Part model, mm, in its own coordinate system. A direction names the side the tool comes from. Give positions to 0.01 mm unless a question says otherwise; leave off trailing zeros. Order: outer loops, then holes, each group sorted by start corner. A loop starts at its lowest first (then second) coordinate and runs counter-clockwise, first axis right, second up. Notation, with made-up numbers: (-15, 48) -> (37, 48) arc R16 cw to (37, 71) -> close; hole circle Ø4 at (65, 25). An arc over 180 degrees is marked (long way). Write item = value, one per line. Start each with the question number.
Item 1: Band-saw the part on C-C on z = 22.5. Write the cut outline in (x, y).
Item 2: Band-saw the part on D-D on x = 13. Write the cut outline in (y, z), plus the area to 3 significant figures.
Item 3: Band-saw the part on A-A on x = 0. Write the cut outline in (y, z), plus the area to 3 significant figures.
Item 4: Tool access for faces 4 (the face through (9, 20, -12)), 5 (the face through (-18, -18.5, 24)): list every direction of +Z, -Z, +X, -X, +Y, -Y with a clear straight run to the whole face (end or side of a thin tool).
Item 5: Band-saw the part on B-B on y = 0. Write the cut outline in (x, z).
Item 6: Drill centre lines: line 1 along Y through (x, z) = (0, -14); line 2 along Y through (x, z) = (0, -6.25); line 3 along X through (y, z) = (-7.5, 19.5). Where is each one in solid material? Low to high.
Item 7: Flat gauge pins, fed straight in: P1, Ø6, axis at x = -2, y = 9.5, coming from the +Z side; P2, Ø4.5, axis at x = -16, z = 5, coming from the -Y side; P3, Ø9.5, axis at x = 0, y = -24, coming from the -Z side. Where does each tip first touch, or does it go through?
Item 8: Pull direction X, two halves, no side cores. Call faces 1 (the face through (0.1, -27.4, -10)), 2 (the face through (9, -20, -12)), 3 (the face through (-27, -16, -12)): +X half, -X half, draft (parallel to the pull), parting line (faces both ways), or undercut.
```python
from build123d import *

# Parameters (mm, degrees)
SKETCH1_R                = 9
SKETCH1_R_2              = 3
SKETCH1_W                = 32
SKETCH1_H                = 8
BOSS_EXTRUDE1_DEPTH      = 25
BOSS_EXTRUDE2_DEPTH      = 15
BOSS_EXTRUDE3_DEPTH      = 14
SKETCH3_R                = 12.5
BOSS_EXTRUDE4_DEPTH      = 20
BOSS_EXTRUDE5_DEPTH      = 18
SKETCH5_R                = 10
BOSS_EXTRUDE6_DEPTH      = 25
BOSS_EXTRUDE7_REACH      = 103.681
BOSS_EXTRUDE7_END_RADIUS = 10
SKETCH7_W                = 5
SKETCH7_H                = 1
BOSS_EXTRUDE8_DEPTH      = 1
SKETCH7_4_W              = 5
SKETCH7_4_H              = 1
BOSS_EXTRUDE9_DEPTH      = 4
SKETCH10_R               = 8
CUT_EXTRUDE1_DEPTH       = 15


with BuildPart() as part:
    # Sketch1 → Boss-Extrude1 (new body)
    # profile 1 of 4: a face of its own
    with BuildSketch(Plane(origin=(0, 0, 0), x_dir=(0, 1, 0), z_dir=(0, 0, 1))):
        with Locations((-24, 0)):
            Circle(SKETCH1_R)
        with Locations(Location((-24, 0, 0), (0, 0, 270))):
            Circle(SKETCH1_R_2, mode=Mode.SUBTRACT)
    # profile 2 of 4: a face of its own
    with BuildSketch(Plane(origin=(0, 0, 0), x_dir=(0, 1, 0), z_dir=(0, 0, 1))):
        with BuildLine():
            ThreePointArc((-15, 0), (-17.636038969, -6.363961031), (-24, -9))
            Line((-24, -9), (-16, -9))
            Line((-16, -9), (16, -9))
            Line((16, -9), (24, -9))
            ThreePointArc((24, -9), (15, 0), (24, 9))
            Line((24, 9), (24, 21))
            Line((24, 21), (8, 33))
            Line((8, 33), (-8, 33))
            Line((-8, 33), (-24, 21))
            Line((-24, 21), (-24, 9))
            ThreePointArc((-24, 9), (-17.636038969, 6.363961031), (-15, 0))
        make_face()
    # profile 3 of 4: a face of its own
    with BuildSketch(Plane(origin=(0, 0, 0), x_dir=(0, 1, 0), z_dir=(0, 0, 1))):
        with Locations((24, 0)):
            Circle(SKETCH1_R)
        with Locations(Location((24, 0, 0), (0, 0, 270))):
            Circle(SKETCH1_R_2, mode=Mode.SUBTRACT)
    # profile 4 of 4: a face of its own
    with BuildSketch(Plane(origin=(0, 0, 0), x_dir=(0, 1, 0), z_dir=(0, 0, 1))):
        with Locations((0, -13)):
            Rectangle(SKETCH1_W, SKETCH1_H)
    extrude(amount=-BOSS_EXTRUDE1_DEPTH)

    # Sketch2 → Boss-Extrude2 (add)
    with BuildSketch(Plane.XY):
        with BuildLine():
            ThreePointArc((-22.5, -13.257073584), (-18, -14), (-13.5, -13.257073584))
            ThreePointArc((-13.5, -13.257073584), (-4, 0), (-13.5, 13.257073584))
            ThreePointArc((-13.5, 13.257073584), (-18, 14), (-22.5, 13.257073584))
            ThreePointArc((-22.5, 13.257073584), (-32, 0), (-22.5, -13.257073584))
        make_face()
    extrude(amount=BOSS_EXTRUDE2_DEPTH)

    # Sketch2<3> → Boss-Extrude3 (add)
    with BuildSketch(Plane.XY):
        with BuildLine():
            ThreePointArc((-22.5, -13.257073584), (-18, -14), (-13.5, -13.257073584))
            Line((-13.5, -13.257073584), (-13.5, -20.257073584))
            Line((-13.5, -20.257073584), (-22.5, -20.257073584))
            Line((-22.5, -20.257073584), (-22.5, -13.257073584))
        make_face()
        with BuildLine():
            Line((-22.5, 20.257073584), (-22.5, 13.257073584))
            ThreePointArc((-22.5, 13.257073584), (-18, 14), (-13.5, 13.257073584))
            Line((-13.5, 13.257073584), (-13.5, 20.257073584))
            Line((-13.5, 20.257073584), (-22.5, 20.257073584))
        make_face()
    extrude(amount=BOSS_EXTRUDE3_DEPTH)

    # Sketch3 → Boss-Extrude4 (add)
    with BuildSketch(Plane.XY.offset(15)):
        with Locations((-18, 0)):
            Circle(SKETCH3_R)
    extrude(amount=BOSS_EXTRUDE4_DEPTH)

    # Sketch3<3> → Boss-Extrude5 (add)
    with BuildSketch(Plane.XY.offset(15)):
        with BuildLine():
            Line((-18, 18.5), (-18, 12.5))
            ThreePointArc((-18, 12.5), (-16.488918226, 12.408329133), (-15, 12.1346611))
            Line((-15, 12.1346611), (-15, 18.5))
            Line((-15, 18.5), (-18, 18.5))
        make_face()
        with BuildLine():
            Line((-15, -18.5), (-15, -12.1346611))
            ThreePointArc((-15, -12.1346611), (-18, -12.5), (-21, -12.1346611))
            Line((-21, -12.1346611), (-21, -18.5))
            Line((-21, -18.5), (-15, -18.5))
        make_face()
    extrude(amount=BOSS_EXTRUDE5_DEPTH)

    # Sketch5 → Boss-Extrude6 (add)
    with BuildSketch(Plane.XY.offset(35)):
        with Locations((-18, 0)):
            Circle(SKETCH5_R)
    extrude(amount=BOSS_EXTRUDE6_DEPTH)

    # Boss-Extrude7: up to this cylinder (the profile starts outside it)
    boss_extrude7_end = Plane(origin=(-18, 0, 55.5), z_dir=(0, 0, -1)) * Cylinder(BOSS_EXTRUDE7_END_RADIUS, 232.362, mode=Mode.PRIVATE)
    # Sketch7 → Boss-Extrude7 (add, up to the surface)
    with BuildSketch(Plane(origin=(-28, 0, 60), x_dir=(0, 0, 1), z_dir=(-1, 0, 0)), mode=Mode.PRIVATE) as boss_extrude7_sk1:
        Polygon((-5, -1), (-5, 0), (-5, 1), (-5, 3), (-8, 3), (-8, -3), (-5, -3), align=None)
    boss_extrude7_tool1 = extrude(boss_extrude7_sk1.sketch, amount=-BOSS_EXTRUDE7_REACH, mode=Mode.PRIVATE) - boss_extrude7_end
    add(boss_extrude7_tool1.solids().sort_by_distance((-28, 0, 53.5))[0])
    add(boss_extrude7_tool1.solids().sort_by_distance((-28, 0, 53.5))[1])
    # Sketch7 → Boss-Extrude7 (add, up to the surface)
    with BuildSketch(Plane(origin=(-28, 0, 60), x_dir=(0, 0, 1), z_dir=(-1, 0, 0)), mode=Mode.PRIVATE) as boss_extrude7_sk2:
        with Locations((-2.5, 0.5)):
            Rectangle(SKETCH7_W, SKETCH7_H)
    boss_extrude7_tool2 = extrude(boss_extrude7_sk2.sketch, amount=-BOSS_EXTRUDE7_REACH, mode=Mode.PRIVATE) - boss_extrude7_end
    add(boss_extrude7_tool2.solids().sort_by_distance((-28, 0.5, 57.5))[0])
    # Sketch7 → Boss-Extrude7 (add, up to the surface)
    with BuildSketch(Plane(origin=(-28, 0, 60), x_dir=(0, 0, 1), z_dir=(-1, 0, 0)), mode=Mode.PRIVATE) as boss_extrude7_sk3:
        with Locations((-2.5, -0.5)):
            Rectangle(SKETCH7_W, SKETCH7_H)
    boss_extrude7_tool3 = extrude(boss_extrude7_sk3.sketch, amount=-BOSS_EXTRUDE7_REACH, mode=Mode.PRIVATE) - boss_extrude7_end
    add(boss_extrude7_tool3.solids().sort_by_distance((-28, -0.5, 57.5))[0])

    # Sketch7<2> → Boss-Extrude8 (add)
    with BuildSketch(Plane(origin=(-28, 0, 60), x_dir=(0, 0, 1), z_dir=(-1, 0, 0))):
        Polygon((-8, -3), (-5, -3), (-5, -1), (-5, 1), (-5, 3), (-8, 3), align=None)
    extrude(amount=BOSS_EXTRUDE8_DEPTH)

    # Sketch7<4> → Boss-Extrude9 (add)
    with BuildSketch(Plane(origin=(-28, 0, 60), x_dir=(0, 0, 1), z_dir=(-1, 0, 0))):
        with Locations((-2.5, 0.5)):
            Rectangle(SKETCH7_4_W, SKETCH7_4_H)
        with Locations((-2.5, -0.5)):
            Rectangle(SKETCH7_4_W, SKETCH7_4_H)
    extrude(amount=BOSS_EXTRUDE9_DEPTH)

    # Sketch10 → Cut-Extrude1 (cut)
    with BuildSketch(Plane(origin=(0, 0, -25), x_dir=(1, 0, 0), z_dir=(0, 0, -1))):
        with Locations(Location((0, 24, 0), (0, 0, 180))):
            Circle(SKETCH10_R)
        with Locations(Location((0, -24, 0), (0, 0, 180))):
            Circle(SKETCH10_R)
    extrude(amount=-CUT_EXTRUDE1_DEPTH, mode=Mode.SUBTRACT)


solid = part.part
```
Values found:
q1.outline = (-21, -18.5) -> (-15, -18.5) -> (-15, -12.13) arc R12.5 ccw to (-15, 12.13) -> (-15, 18.5) -> (-18, 18.5) -> (-18, 12.5) arc R12.5 ccw to (-21, -12.13) -> close
q2.outline = (-16, -25) -> (16, -25) -> (16, 0) -> (-16, 0) -> close
q2.area = 800 mm^2
q3.outline = (-33, -25) -> (-32, -25) -> (-32, -10) -> (-27, -10) -> (-27, 0) -> (-33, 0) -> close; (-21, -10) -> (-16, -10) -> (-16, -25) -> (16, -25) -> (16, -10) -> (21, -10) -> (21, 0) -> (-21, 0) -> close; (27, -10) -> (32, -10) -> (32, -25) -> (33, -25) -> (33, 0) -> (27, 0) -> close
q3.area = 1,050 mm^2
q4.face_4 = +Z, -Z, +X, +Y
q4.face_5 = +Z, +X, -X, -Y
q5.outline = (-33, -25) -> (17, -25) -> (17, 0) -> (-4, 0) -> (-4, 15) -> (-5.5, 15) -> (-5.5, 35) -> (-8, 35) -> (-8, 60) -> (-32, 60) -> (-32, 55) -> (-29, 55) -> (-29, 52) -> (-28, 52) -> (-28, 35) -> (-30.5, 35) -> (-30.5, 15) -> (-32, 15) -> (-32, 0) -> (-33, 0) -> close
q6.line_1 = -33 to -32, -16 to 16, 32 to 33
q6.line_2 = -33 to -27, -21 to 21, 27 to 33
q6.line_3 = -28 to -8
q7.P1 = 0
q7.P2 = -20.26
q7.P3 = -10
q8.face_1 = undercut
q8.face_2 = +X half
q8.face_3 = -X half
